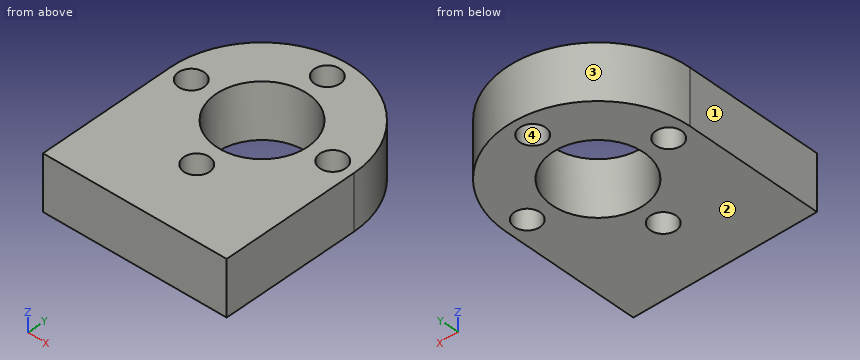
from build123d import *

# Parameters (mm, degrees)
SKETCH1_R           = 12.7
BOSS_EXTRUDE1_DEPTH = 7.62
SKETCH2_R           = 6.35
CUT_EXTRUDE1_DEPTH  = 7.62
SKETCH3_R           = 1.778
CUT_EXTRUDE2_DEPTH  = 7.62
CIRPATTERN1_COUNT   = 4


with BuildPart() as part:
    # Sketch1 → Boss-Extrude1 (new body)
    with BuildSketch(Plane.XY):
        with BuildLine():
            Line((0, -31.75), (0, -12.7))
            ThreePointArc((0, -12.7), (-12.699999961, -25.4), (-25.4, -12.700000079))
            Line((-25.4, -12.700000079), (-25.4, -31.75))
            Line((-25.4, -31.75), (0, -31.75))
        make_face()
        with Locations((-12.7, -12.7)):
            Circle(SKETCH1_R)
    extrude(amount=BOSS_EXTRUDE1_DEPTH)

    # Sketch2 → Cut-Extrude1 (cut)
    with BuildSketch(Plane.XY.offset(7.62)):
        with Locations((-12.7, -12.7)):
            Circle(SKETCH2_R)
    extrude(amount=-CUT_EXTRUDE1_DEPTH, mode=Mode.SUBTRACT)

    # Sketch3 → Cut-Extrude2 (cut)
    with BuildSketch(Plane.XY.offset(7.62)):
        with Locations((-12.7, -2.921)):
            Circle(SKETCH3_R)
    cut_extrude2 = extrude(amount=-CUT_EXTRUDE2_DEPTH, mode=Mode.SUBTRACT)

    # CirPattern1: Cut-Extrude2 ×4 about axis
    cirpattern1_axis = Axis((-12.7, -12.7, 0), (0, 0, 1))
    for i in range(1, CIRPATTERN1_COUNT):
        add(cut_extrude2.rotate(cirpattern1_axis, i * 360 / CIRPATTERN1_COUNT), mode=Mode.SUBTRACT)


solid = part.part
Can you work these out from the model? Positions are in its coordinate system, mm. Face numbers are marked on the shaded views. Coordinates: 2 decimals unless noted, no trailing zeros. Order: outer loops, then holes, each group sorted by start corner. A loop starts at its lowest first (then second) coordinate and runs counter-clockwise, first axis right, second up. Notation, with made-up numbers: (85, 73.5) -> (111, 73.5) arc R28 ccw to (111, 106.5) -> close; hole circle Ø4 at (-26.5, 13.25). An arc over 180 degrees is marked (long way). Use one line per item in the form item = value.
Q1. Will these pins go through, and if not, where does the flat tip stop? P1, Ø1, axis at x = -11, y = -9, coming from the +Z side; P2, Ø12, axis at x = -9.5, y = -18, coming from the +Z side; P3, Ø1, axis at x = -18, z = 6, coming from the +Y side; P4, Ø2, axis at x = -14.5, z = 3.5, coming from the +Y side.
From the geometry:
P1 = through
P2 = 7.62
P3 = -0.94
P4 = -0.03
Q2. I need wall thicknesses on L1, parallel to Y at x = -12.7, z = 5.75; L2, parallel to Y at x = -13.75, z = 3; L3, parallel to X at y = -24, z = 4. Which ranges of each line are inside material? Lowest first, please.
From the geometry:
L1 = -31.75 to -24.26, -20.7 to -19.05, -6.35 to -4.7, -1.14 to 0
L2 = -31.75 to -23.91, -21.04 to -18.96, -6.44 to -4.36, -1.49 to -0.04
L3 = -25.4 to -13.62, -11.78 to 0
Q3. Imagine slicing it at A-A, the plane x = -12.7. List the corners of the cut face in (y, z) for me, then the cut area to 3 significant figures.
From the geometry:
outline = (-31.75, 0) -> (-24.26, 0) -> (-24.26, 7.62) -> (-31.75, 7.62) -> close; (-20.7, 0) -> (-19.05, 0) -> (-19.05, 7.62) -> (-20.7, 7.62) -> close; (-6.35, 0) -> (-4.7, 0) -> (-4.7, 7.62) -> (-6.35, 7.62) -> close; (-1.14, 0) -> (0, 0) -> (0, 7.62) -> (-1.14, 7.62) -> close
area = 91.0 mm²
Q4. Imagine slicing it at C-C, the plane y = -10. List the corners of the cut face in (x, z) for me, then the cut area to 3 significant figures.
From the geometry:
outline = (-25.11, 0) -> (-18.45, 0) -> (-18.45, 7.62) -> (-25.11, 7.62) -> close; (-6.95, 0) -> (-0.29, 0) -> (-0.29, 7.62) -> (-6.95, 7.62) -> close
area = 102 mm²
Q5. Imagine slicing it at D-D, the plane z = 1.25. List the corners of the cut face in (x, y) for me, then the cut area to 3 significant figures.
From the geometry:
outline = (-25.4, -31.75) -> (0, -31.75) -> (0, -12.7) arc R12.7 ccw to (-25.4, -12.7) -> close; hole circle Ø3.56 at (-22.48, -12.7); hole circle Ø12.7 at (-12.7, -12.7); hole circle Ø3.56 at (-12.7, -22.48); hole circle Ø3.56 at (-12.7, -2.92); hole circle Ø3.56 at (-2.92, -12.7)
area = 571 mm²
Q6. We'd pull the mould along X, two halves only. Please class the marked faces 1, 2, 3 and 4: released by +X, released by -X, zero draft, split by the parting line, or undercut.
From the geometry:
face_1 = released by -X
face_2 = zero draft
face_3 = split by the parting line
face_4 = undercut
Q7. Imagine slicing it at B-B, the plane x = -4. List the corners of the cut face in (y, z) for me.
From the geometry:
outline = (-31.75, 0) -> (-14.11, 0) -> (-14.11, 7.62) -> (-31.75, 7.62) -> close; (-11.29, 0) -> (-3.45, 0) -> (-3.45, 7.62) -> (-11.29, 7.62) -> close
